Geometry: final body of the model. Coordinates: model frame, mm. Face numbers are marked on the shaded views. A direction names the side the tool comes from. Coordinates: 2 decimals unless noted, no trailing zeros. Order: outer loops, then holes, each group sorted by start corner. A loop starts at its lowest first (then second) coordinate and runs counter-clockwise, first axis right, second up. Notation, with made-up numbers: M 22,29.5 L 54,29.5 A6 cw 54,36.5 Z; hole C -4.75,-34.75 d4. An arc over 180 degrees is marked long. Use CSV: the item, a comma, the result in double quotes. Start each with the question number.
Q1. Ray query, probe 1 along Z at (x, y) = (-1, 23.5); probe 2 along X at (y, z) = (32, 12.25); probe 3 along Y at (x, z) = (0.5, 12.75). Return the intervals inside material, ascending.
Q2. Section query C-C, the plane z = 15.5. Output: boundary loops of the cut face in (x, y), and give its area (3 significant figures).
Q3. Access query for the marked faces 1, 2 and 3. Directions: +Z, -Z, +X, -X, +Y, -Y. A direction counts if a zero-diameter tool reaches every point of the face in a straight line with its end or side. Return the directions, or none.
Q4. First-contact query: P1, Ø4, axis at x = -2, z = 7.5, coming from the -Y side; P2, Ø10, axis at y = 29.5, z = 8, coming from the +X side; P3, Ø1, axis at x = 2.5, z = 21.5, coming from the -Y side. Flat tips, straight axial feed; report the tip coordinate or a pass-through.
Q5. Section query B-B, the plane y = 29. Output: boundary loops of the cut face in (x, z), and give its area (3 significant figures).
Q6. Section query A-A, the plane z = 11. Output: boundary loops of the cut face in (x, y), and give its area (3 significant figures).
Q7. Mould query, pull axis Y, two halves, no side actions, for the marked faces 4, 5 and 6. Classes: +Y half, -Y half, draft (parallel to the pull), parting line (faces both ways), or undercut.
from build123d import *

# Parameters (mm, degrees)
RESSALTO_EXTRUS_O1_DEPTH = 22
RESSALTO_EXTRUS_O2_DEPTH = 16
FILETE1_R                = 5
FILETE2_R                = 0.5
FILETE3_R                = 0.5
CORTE_EXTRUS_O1_DEPTH    = 43.143081298


with BuildPart() as part:
    # Esboço2 → Ressalto-extrusão1 (new body)
    with BuildSketch(Plane.XY):
        Polygon((-1.5, 34.66683278), (1.5, 34.66683278), (1.5, 11.46683278), (8, 6.46683278), (8, 3.46683278), (-8, 3.46683278), (-8, 6.46683278), (-1.5, 11.46683278), align=None)
    extrude(amount=RESSALTO_EXTRUS_O1_DEPTH)

    # Esboço3 → Ressalto-extrusão2 (add)
    with BuildSketch(Plane(origin=(8, 0, 0), x_dir=(0, 0, -1), z_dir=(1, 0, 0))):
        with BuildLine():
            Line((-18.5, 3.46683278), (-3.5, 3.46683278))
            ThreePointArc((-3.5, 3.46683278), (-11, 0.913484582), (-18.5, 3.46683278))
        make_face()
    extrude(amount=-RESSALTO_EXTRUS_O2_DEPTH)

    # Filete1
    filete1_edges = [part.edges().sort_by_distance(p)[0] for p in [
        (0, 3.46683278, 3.5),
        (0, 3.46683278, 18.5),
    ]]
    fillet(filete1_edges, radius=FILETE1_R)

    # Filete2
    filete2_edges = [part.edges().sort_by_distance(p)[0] for p in [
        (0, 34.66683278, 22),
        (1.5, 23.06683278, 0),
        (4.75, 8.96683278, 0),
        (-1.5, 23.06683278, 22),
        (8, 6.46683278, 11),
        (-1.5, 11.46683278, 11),
        (-1.5, 34.66683278, 11),
        (1.5, 34.66683278, 11),
        (-4.75, 8.96683278, 22),
        (-8, 4.96683278, 22),
        (8, 4.96683278, 22),
        (4.75, 8.96683278, 22),
        (1.5, 23.06683278, 22),
        (8, 4.96683278, 0),
        (-8, 4.96683278, 0),
        (-4.75, 8.96683278, 0),
        (-1.5, 23.06683278, 0),
        (0, 34.66683278, 0),
    ]]
    fillet(filete2_edges, radius=FILETE2_R)

    # Filete3
    filete3_edges = [part.edges().sort_by_distance(p)[0] for p in [
        (-8, 6.46683278, 11),
        (-7.843873382, 6.389955799, 21.86297534),
        (-7.843873382, 6.389955799, 0.13702466),
    ]]
    fillet(filete3_edges, radius=FILETE3_R)

    # Esboço4 → Corte-extrusão1 (cut, through all)
    with BuildSketch(Plane(origin=(1.5, 0, 0), x_dir=(0, 0, -1), z_dir=(1, 0, 0))):
        with BuildLine():
            Line((-14, 27.885318181), (-14, 21.885318181))
            ThreePointArc((-14, 21.885318181), (-11, 19.91907546), (-8, 21.885318181))
            Line((-8, 21.885318181), (-8, 27.885318181))
            ThreePointArc((-8, 27.885318181), (-11, 30.885318181), (-14, 27.885318181))
        make_face()
    extrude(amount=-CORTE_EXTRUS_O1_DEPTH, mode=Mode.SUBTRACT)


solid = part.part
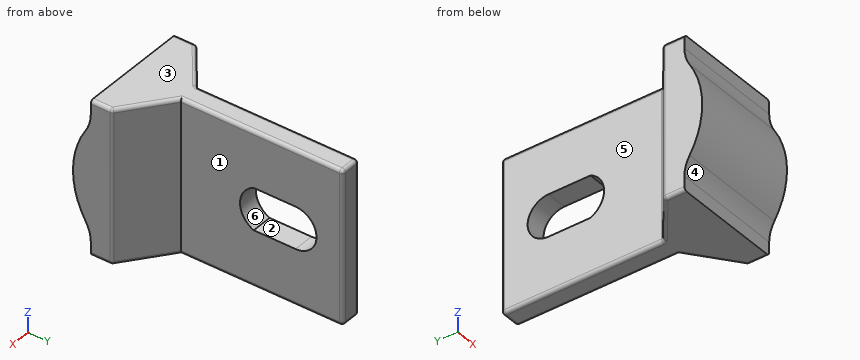
Responses:
1,probe 1,"z = 0 to 8, 14 to 22"
1,probe 2,"x = -1.5 to 1.5"
1,probe 3,"y = 1.04 to 20.43, 30.32 to 34.67"
2,outline,"M -8,1.77 L 8,1.77 L 8,6.22 A0.5 ccw 7.8,6.62 L 1.5,11.47 L 1.5,34.17 A0.5 ccw 1,34.67 L -1,34.67 A0.5 ccw -1.5,34.17 L -1.5,11.71 A0.5 cw -1.7,11.32 L -7.8,6.62 A0.5 ccw -8,6.22 Z"
2,area,"192 mm²"
3,face 1,"+Z, -Z, +X, +Y"
3,face 2,"+X, -X"
3,face 3,"+Z, +X, -X, +Y, -Y"
4,P1,"stops at y = 1.01"
4,P2,"stops at x = 1.5"
4,P3,"stops at y = 3.47"
5,outline,"M -1.5,0.5 A0.5 ccw -1,0 L 1,0 A0.5 ccw 1.5,0.5 L 1.5,8.21 L -1.5,8.21 Z; M -1.5,13.79 L 1.5,13.79 L 1.5,21.5 A0.5 ccw 1,22 L -1,22 A0.5 ccw -1.5,21.5 Z"
5,area,"49.1 mm²"
6,outline,"M -8,0.91 L 8,0.91 L 8,6.22 A0.5 ccw 7.8,6.62 L 1.5,11.47 L 1.5,19.92 L -1.5,19.92 L -1.5,11.71 A0.5 cw -1.7,11.32 L -7.8,6.62 A0.5 ccw -8,6.22 Z; M -1.5,30.89 L 1.5,30.89 L 1.5,34.17 A0.5 ccw 1,34.67 L -1,34.67 A0.5 ccw -1.5,34.17 Z"
6,area,"173 mm²"
7,face 4,"-Y half"
7,face 5,"draft"
7,face 6,"undercut"
